Print and shaded views of the part. All mm, measured from the part's lowest x, y and z. A direction names the side the tool comes from. Round coordinates to 2 decimals unless told otherwise and drop trailing zeros. Loops run counter-clockwise (first coordinate to the right, second up) from the corner with the lowest first, then second, coordinate; pieces in that order, holes last. Notation, with made-up numbers: (54.5, 14) - (77.5, 14) arc R19 ccw to (77.5, 45) - close; hole circle Ø1 at (67, -13). An arc over 180 degrees is marked (long way). Answer as a JSON object with one key per item and string values.
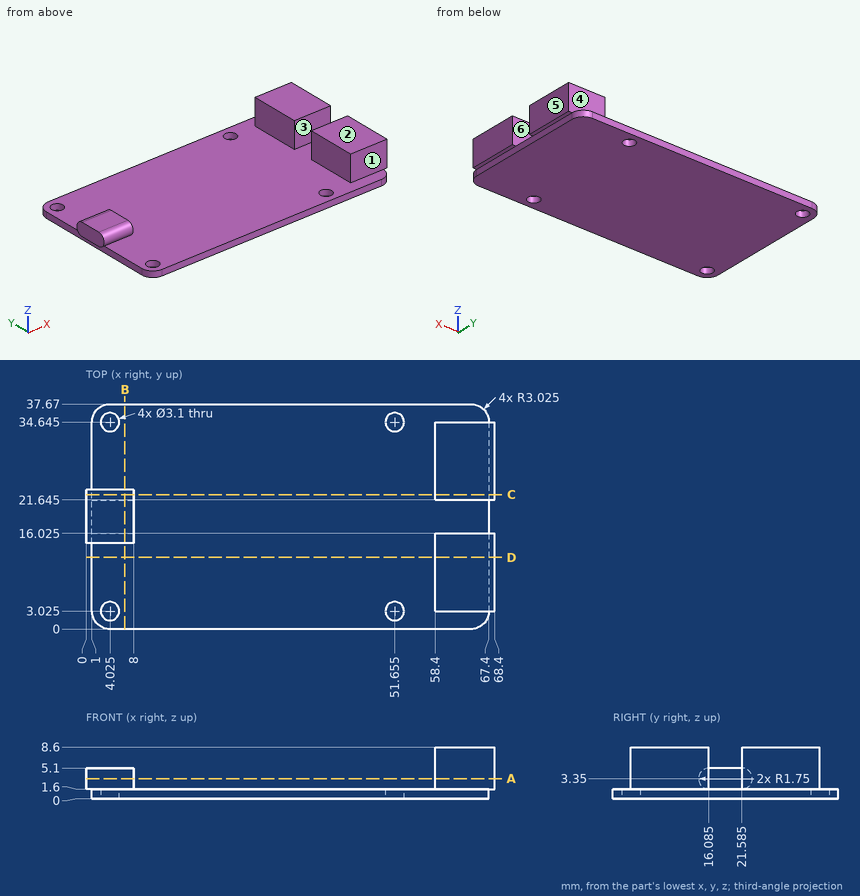
1) Slice it at D-D on y = 12. List the corners of the cut face in (x, z), then the cut area to 3 significant figures.
Values follow:
{"outline": "(1, 0) - (67.4, 0) - (67.4, 1.6) - (68.4, 1.6) - (68.4, 8.6) - (58.4, 8.6) - (58.4, 1.6) - (1, 1.6) - close", "area": "176 mm²"}
2) Tool access for the marked faces 1, 2 and 3: list every direction of +Z, -Z, +X, -X, +Y, -Y with a clear straight run to the whole face (end or side of a thin tool).
Values follow:
{"face 1": "+Z, +X, -X, -Y", "face 2": "+Z, +X, -X, +Y, -Y", "face 3": "+Z, +X"}
3) Drop flat-ended pins along their axis: P1, Ø5, axis at x = 15, y = 9, coming from the -Z side; P2, Ø1, axis at x = 40.5, y = 7.5, coming from the +Z side; P3, Ø0.8, axis at x = 0.5, y = 17.5, coming from the -Z side; P4, Ø1.3, axis at y = 25.5, z = 0.5, coming from the +X side. Give the stop position or say it passes through.
Values follow:
{"P1": "z = 0", "P2": "z = 1.6", "P3": "z = 1.6", "P4": "x = 67.4"}
4) Slice it at A-A on z = 3.35. List the corners of the cut face in (x, y) (3 decimals).
Values follow:
{"outline": "(0, 14.335) - (8, 14.335) - (8, 23.335) - (0, 23.335) - close; (58.4, 3.025) - (68.4, 3.025) - (68.4, 16.025) - (58.4, 16.025) - close; (58.4, 21.645) - (68.4, 21.645) - (68.4, 34.645) - (58.4, 34.645) - close"}
5) Slice it at C-C on y = 22.5. List the corners of the cut face in (x, z).
Values follow:
{"outline": "(0, 1.86) - (8, 1.86) - (8, 4.84) - (0, 4.84) - close; (1, 0) - (67.4, 0) - (67.4, 1.6) - (68.4, 1.6) - (68.4, 8.6) - (58.4, 8.6) - (58.4, 1.6) - (1, 1.6) - close"}
6) Slice it at B-B on x = 6.5. List the corners of the cut face in (y, z) (3 decimals).
Values follow:
{"outline": "(0, 0) - (37.67, 0) - (37.67, 1.6) - (21.585, 1.6) arc R1.75 ccw to (21.585, 5.1) - (16.085, 5.1) arc R1.75 ccw to (16.085, 1.6) - (0, 1.6) - close"}
7) Probe probe 1 along Y at (x, z) = (65, 4) (3 decimals); probe 2 along Z at (x, y) = (54, 10.5); probe 3 along X at (y, z) = (11, 7.75). List the from-to ranges inside material, lowest first.
Values follow:
{"probe 1": "3.025 to 16.025, 21.645 to 34.645", "probe 2": "0 to 1.6", "probe 3": "58.4 to 68.4"}
8) Two-plate mould, pull along Y, no slides. Class the marked faces 4, 5 and 6: pulls with the +Y half, pulls with the -Y half, needs draft (parallel to the pull), parting line crosses it, or undercut.
Values follow:
{"face 4": "pulls with the +Y half", "face 5": "needs draft", "face 6": "undercut"}
